Autodesk Inventor part; units mm, degrees
ref_plane "YZ Plane" through (0, 0, 0) normal (1, 0, 0) x (0, 1, 0)
ref_plane "XZ Plane" through (0, 0, 0) normal (0, 1, 0) x (-1, 0, 0)
ref_plane "XY Plane" through (0, 0, 0) normal (0, 0, 1) x (1, 0, 0)
sketch "Sketch1" plane through (0, 0, 0) normal (0, 0, 1) x (1, 0, 0)
  circle A0 centre (0, 0) radius 13.8
  circle A1 centre (0, 0) radius 11.5
  circle A2 centre (0, 0) radius 15.6
  circle A3 centre (0, 0) radius 12.5
  dimension "d0" = 27.6
  dimension "d1" = 23
  dimension "d2" = 31.2
  dimension "d3" = 25
extrude "Extrusion1" add sketch "Sketch1" along normal blind 1 contours A3
extrude "Extrusion2" add sketch "Sketch1" along normal blind 4 contours A0
sketch "Sketch2" plane through (0, 0, 4) normal (0, 0, 1) x (1, 0, 0)
  circle A0 centre (0, 0) radius 15.6
  circle A1 centre (0, 0) radius 12.5
extrude "Extrusion3" add sketch "Sketch2" along normal blind 1.5
sketch "Sketch3" plane through (0, 0, 5.5) normal (0, 0, 1) x (1, 0, 0)
  line L0 (0.5, 8.5) -> (-0.5, 8.5)
  line L1 (-0.5, 8.5) -> (-0.5, 16.5)
  line L2 (-0.5, 16.5) -> (0.5, 16.5)
  line L3 (0.5, 16.5) -> (0.5, 8.5)
  circle A0 centre (0, 0) radius 12.5
  line L4 (0.5, 8.5) -> (-0.5, 16.5) construction
  line L5 (-0.5, 8.5) -> (0.5, 16.5) construction
  point P0 (0, 12.5)
  dimension "d10" = 1
  dimension "d11" = 8
extrude "Extrusion4" cut sketch "Sketch3" against normal blind 10 contours L0 L1 A0 L3 | A0 L1 L2 L3 picked at (0.0556, 9.833)
properties part number "25mmFilterAdapter"
Build history of the part. All positions in model axes, mm. A direction names the side the tool comes from. Coordinates: 2 decimals unless noted, no trailing zeros. Write each loop counter-clockwise with the first axis right and the second up, starting at its lowest first coordinate (ties: lowest second). Pieces come first, ordered by that corner, then holes.
1. Pull direction Y, two halves, no side cores. Call faces 4 (the flat face through (0.5, 13.6, 3.4)), 5 (the flat face through (-6, -10, 1)): released by +Y, released by -Y, zero draft, split by the parting line, or undercut.
Answer block:
face 4: zero draft
face 5: undercut
2. Band-saw the part on D-D, the plane z = 5.05. Give the cut face in (x, y).
Answer block:
outline: (-0.5, 12.49) - (-0.5, 15.59) arc R15.6 ccw (long way) to (0.5, 15.59) - (0.5, 12.49) arc R12.5 cw (long way) to start
3. Band-saw the part on A-A, the plane x = 0. Give the cut face in (y, z), and give its area (4 significant figures).
Answer block:
outline: (-15.6, 4) - (-13.8, 4) - (-13.8, 0) - (-11.5, 0) - (-11.5, 1) - (-12.5, 1) - (-12.5, 5.5) - (-15.6, 5.5) - close
area: 10.85 mm2
4. Drill centre lines: probe 1 along X at (y, z) = (0, 0.5); probe 2 along X at (y, z) = (0, 4.1); probe 3 along Y at (x, z) = (0, 4.4). Where is each one in solid material? Low to high.
Answer block:
probe 1: x = -13.8 to -11.5, 11.5 to 13.8
probe 2: x = -15.6 to -12.5, 12.5 to 15.6
probe 3: y = -15.6 to -12.5
5. 3-axis set-ups, long thin cutter, end or side, ignore diameter. For faces 1 (the flat face through (-0.5, 13.5, 3.4)), 2 (the flat face through (1, -14, 4)), 3 (the flat face through (-9.3, -7.1, 0)): which of +Z, -Z, +X, -X, +Y, -Y reach the whole face in a straight line?
Answer block:
face 1: +Z, -Z, +Y
face 2: -Z
face 3: -Z, +X, -X, +Y, -Y
6. Band-saw the part on B-B, the plane y = -10.5. Give the cut face in (x, z).
Answer block:
outline: (-11.54, 4) - (-8.95, 4) - (-8.95, 0) - (-4.69, 0) - (-4.69, 1) - (-6.78, 1) - (-6.78, 5.5) - (-11.54, 5.5) - close; (4.69, 0) - (8.95, 0) - (8.95, 4) - (11.54, 4) - (11.54, 5.5) - (6.78, 5.5) - (6.78, 1) - (4.69, 1) - close
7. Band-saw the part on C-C, the plane x = -4. Give the cut face in (y, z).
Answer block:
outline: (-15.08, 4) - (-13.21, 4) - (-13.21, 0) - (-10.78, 0) - (-10.78, 1) - (-11.84, 1) - (-11.84, 5.5) - (-15.08, 5.5) - close; (10.78, 0) - (13.21, 0) - (13.21, 4) - (15.08, 4) - (15.08, 5.5) - (11.84, 5.5) - (11.84, 1) - (10.78, 1) - close
8. Drop flat-ended pins along their axis: pin 1 (8 mm diameter, centred on x = 2.5, y = -2.5, fed in from +Z); pin 2 (2 mm diameter, centred on y = -6.5, z = 1.5, fed in from -X). Give the stop position or say it passes through.
Answer block:
pin 1: passes through
pin 2: stops at x = -12.66
